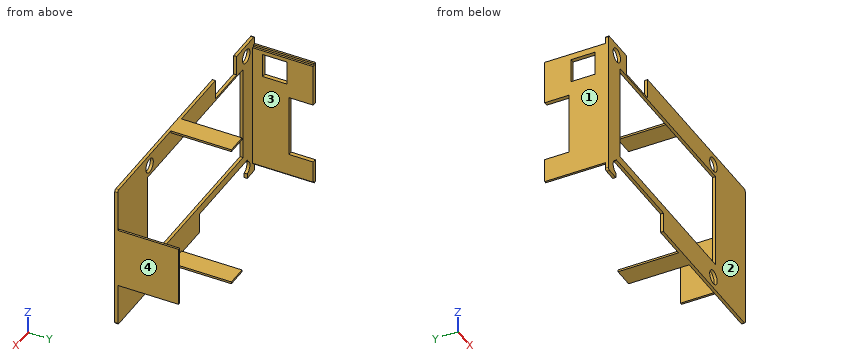
```python
from build123d import *

# Parameters (mm, degrees)
SKETCH_1_W          = 1
SKETCH_1_H          = 1
EXTRUDE_1_DEPTH     = 30
SKETCH_1_5_W        = 129
SKETCH_1_5_H        = 73
EXTRUDE_3_DEPTH     = 1.5
SKETCH_4_W          = 1
SKETCH_4_H          = 30
SKETCH_4_W_2        = 10
SKETCH_4_H_2        = 1
EXTRUDE_4_DEPTH     = 30
SKETCH_8_W          = 31
SKETCH_8_H          = 12
SKETCH_8_W_2        = 12
CUT_EXTRUDE_5_DEPTH = 2
SKETCH_6_W          = 90
SKETCH_6_H          = 48
SKETCH_6_W_2        = 20
SKETCH_6_H_2        = 10
SKETCH_6_W_3        = 45
CUT_EXTRUDE_6_DEPTH = 2
FILLET_1_R          = 1
FILLET_6_R          = 1
FILLET_7_R          = 1
SKETCH_10_R         = 3.5
CUT_EXTRUDE_7_DEPTH = 2


with BuildPart() as part:
    # Sketch 1 → Extrude 1 (new body)
    with BuildSketch(Plane(origin=(0, 0, 0), x_dir=(1, 0, 0), z_dir=(0, 1, 0))):
        with Locations((-64, -32)):
            Rectangle(SKETCH_1_W, SKETCH_1_H)
        Polygon((-63.5, 31.5), (-64.5, 31.5), (-64.5, -31.5), (-63.5, -31.5), (-62.5, -31.5), (-62.5, 31.5), align=None)
        with Locations((-64, 32)):
            Rectangle(SKETCH_1_W, SKETCH_1_H)
    extrude(amount=EXTRUDE_1_DEPTH)

    # Sketch 1_5 → Extrude 3 (add)
    with BuildSketch(Plane(origin=(0, 0, 0), x_dir=(1, 0, 0), z_dir=(0, 1, 0))):
        Rectangle(SKETCH_1_5_W, SKETCH_1_5_H)
    extrude(amount=-EXTRUDE_3_DEPTH)

    # Sketch 4 → Extrude 4 (add)
    with BuildSketch(Plane(origin=(0, 0, 0), x_dir=(1, 0, 0), z_dir=(0, 1, 0))):
        with Locations((64, 0)):
            Rectangle(SKETCH_4_W, SKETCH_4_H)
        with Locations((9.5, -36)):
            Rectangle(SKETCH_4_W_2, SKETCH_4_H_2)
        with Locations((9.5, 36)):
            Rectangle(SKETCH_4_W_2, SKETCH_4_H_2)
    extrude(amount=EXTRUDE_4_DEPTH)

    # Sketch 8 → Cut-Extrude 5 (cut)
    with BuildSketch(Plane.ZY.offset(64.5)):
        with Locations((-5, 24)):
            Rectangle(SKETCH_8_W, SKETCH_8_H)
        with Locations((23.5, 11)):
            Rectangle(SKETCH_8_W_2, SKETCH_8_H)
    extrude(amount=-CUT_EXTRUDE_5_DEPTH, mode=Mode.SUBTRACT)

    # Sketch 6 → Cut-Extrude 6 (cut)
    with BuildSketch(Plane.XZ.offset(1.5)):
        with Locations((-8.5, 1.5)):
            Rectangle(SKETCH_6_W, SKETCH_6_H)
        with Locations((-37.5, 31.5)):
            Rectangle(SKETCH_6_W_2, SKETCH_6_H_2)
        with Locations((-35, -31.5)):
            Rectangle(SKETCH_6_W_3, SKETCH_6_H_2)
    extrude(amount=-CUT_EXTRUDE_6_DEPTH, mode=Mode.SUBTRACT)

    # Fillet 1
    fillet_1_edges = [part.edges().sort_by_distance(p)[0] for p in [
        (-64.5, -0.75, -36.5),
    ]]
    fillet(fillet_1_edges, radius=FILLET_1_R)

    # Fillet 6
    fillet_6_edges = [part.edges().sort_by_distance(p)[0] for p in [
        (-64.5, -0.75, 36.5),
    ]]
    fillet(fillet_6_edges, radius=FILLET_6_R)

    # Fillet 7
    fillet_7_edges = [part.edges().sort_by_distance(p)[0] for p in [
        (64.5, -0.75, -36.5),
        (64.5, -0.75, 36.5),
    ]]
    fillet(fillet_7_edges, radius=FILLET_7_R)

    # Sketch 10 → Cut-Extrude 7 (cut)
    with BuildSketch(Plane(origin=(0, -1.5, 0), x_dir=(-1, 0, 0), z_dir=(0, -1, 0))):
        with Locations((-34.5, 30.7)):
            Circle(SKETCH_10_R)
        with Locations((-34.5, -30.7)):
            Circle(SKETCH_10_R)
        with Locations((56.5, -30.7)):
            Circle(SKETCH_10_R)
        with BuildLine():
            Line((57.5, 27.345898034), (57.5, 34.054101966))
            ThreePointArc((57.5, 34.054101966), (60, 30.7), (57.5, 27.345898034))
        make_face()
    extrude(amount=-CUT_EXTRUDE_7_DEPTH, mode=Mode.SUBTRACT)


solid = part.part
```
The model under review builds one solid part; all positions refer to its coordinate system, in mm. Face numbers are marked on the shaded views. Round coordinates to 2 decimals unless told otherwise and drop trailing zeros. Order: outer loops, then holes, each group sorted by start corner. A loop starts at its lowest first (then second) coordinate and runs counter-clockwise, first axis right, second up. Notation, with made-up numbers: M -14,43.25 L 22,43.25 A28 ccw 22,80.25 Z; hole C 54.5,8.5 d8. An arc over 180 degrees is marked long. Use a Markdown table: item, result.
1) Consider section B-B (z = 19.5). Write out the cut boundary in (x, y).
Report:
| item | result |
|---|---|
| outline | M -64.5,-1.5 L -53.5,-1.5 L -53.5,0 L -62.5,0 L -62.5,5 L -64.5,5 Z; M -64.5,17 L -62.5,17 L -62.5,30 L -64.5,30 Z; M 36.5,-1.5 L 64.5,-1.5 L 64.5,0 L 36.5,0 Z |
2) Consider section D-D (x = 34.5). Write out the cut boundary in (y, z), then the cut area to 3 significant figures.
Report:
| item | result |
|---|---|
| outline | M -1.5,-36.5 L 0,-36.5 L 0,-34.2 L -1.5,-34.2 Z; M -1.5,-27.2 L 0,-27.2 L 0,-22.5 L -1.5,-22.5 Z; M -1.5,25.5 L 0,25.5 L 0,27.2 L -1.5,27.2 Z; M -1.5,34.2 L 0,34.2 L 0,36.5 L -1.5,36.5 Z |
| area | 16.5 mm^2 |
3) Insertion check: pin 1 (12 mm diameter, centred on x = 2.5, y = 3.5, fed in from +Z); pin 2 (5.5 mm diameter, centred on x = -56.5, z = 30.7, fed in from +Y); pin 3 (1 mm diameter, centred on x = -63.5, z = -2.5, fed in from +Y); pin 4 (0.5 mm diameter, centred on y = 14, z = 32, fed in from +X). Each pin has a flat end and moves straight along its axis. Give the tip position at first contact, or say it passes through.
Report:
| item | result |
|---|---|
| pin 1 | z = 36.5 |
| pin 2 | through |
| pin 3 | y = 18 |
| pin 4 | x = -63.5 |
4) Consider section C-C (x = 16.5). Write out the cut boundary in (y, z).
Report:
| item | result |
|---|---|
| outline | M -1.5,-36.5 L 0,-36.5 L 0,-22.5 L -1.5,-22.5 Z; M -1.5,25.5 L 0,25.5 L 0,36.5 L -1.5,36.5 Z |
5) Consider section A-A (y = 24). Write out the cut boundary in (x, z).
Report:
| item | result |
|---|---|
| outline | M -64.5,-32.5 L -63.5,-32.5 L -63.5,-31.5 L -62.5,-31.5 L -62.5,-20.5 L -64.5,-20.5 Z; M -64.5,10.5 L -62.5,10.5 L -62.5,31.5 L -63.5,31.5 L -63.5,32.5 L -64.5,32.5 Z; M 4.5,-36.5 L 14.5,-36.5 L 14.5,-35.5 L 4.5,-35.5 Z; M 4.5,35.5 L 14.5,35.5 L 14.5,36.5 L 4.5,36.5 Z; M 63.5,-15 L 64.5,-15 L 64.5,15 L 63.5,15 Z |
6) Wall thickness on line 1 along X through (y, z) = (-0.8, 30.7); line 2 along Z through (x, y) = (34.5, -1.05); line 3 along X through (y, z) = (4, -5): over which ranges is each line inside the solid? List them lowest first. Write a range as [from, to].
Report:
| item | result |
|---|---|
| line 1 | [-64.5, -60], [-53, -47.5], [-27.5, 31], [38, 64.5] |
| line 2 | [-36.5, -34.2], [-27.2, -22.5], [25.5, 27.2], [34.2, 36.5] |
| line 3 | [-64.5, -62.5], [63.5, 64.5] |
7) Draft analysis for pull direction X (two halves, no side actions). For the marked faces 1, 2, 3 and 4, state which applies: released by +X, released by -X, zero draft, split by the parting line, or undercut.
Report:
| item | result |
|---|---|
| face 1 | released by -X |
| face 2 | zero draft |
| face 3 | undercut |
| face 4 | released by +X |
